The drawing under review shows one solid part. Ordinate dimensions are in mm from its lowest x, y, z. Round coordinates to 2 decimals unless told otherwise and drop trailing zeros. Order: outer loops, then holes, each group sorted by start corner. A loop starts at its lowest first (then second) coordinate and runs counter-clockwise, first axis right, second up. Notation, with made-up numbers: M 81.5,13 L 139.5,13 A14 cw 139.5,28 Z; hole C -29.5,-25 d5. An arc over 180 degrees is marked long. Answer as a JSON object with one key per item and string values. Group by question number.
1) Consider section D-D, the plane x = 7. Write out the cut boundary in (y, z) (1 decimal).
2) Consider section A-A, the plane x = 70.5. Write out the cut boundary in (y, z).
3) Insertion check: pin 1 Ø4 at (x, z) = (15.5, 69) entering from -Y; pin 2 Ø6.5 at (x, y) = (71.5, 7) entering from +Z; pin 3 Ø2 at (x, y) = (33.5, 3) entering from +Z (1 decimal); pin 4 Ø1 at (x, y) = (8.5, 5) entering from -Z. Each pin has a flat end and moves straight along its axis. Give the tip position at first contact, or say it passes through.
4) To check wall thickness, follow line 1 (Y direction, x = 1.1, z = 70.5); line 2 (Y direction, x = 70.5, z = 1.9); line 3 (Z direction, x = 73.5, y = 8). State the ranges of each line that lie inside material, in increasing order.
5) Consider section C-C, the plane y = 10.25. Write out the cut boundary in (x, z).
6) Consider section B-B, the plane z = 70.5. Write out the cut boundary in (x, y), then the cut area to 3 significant figures.
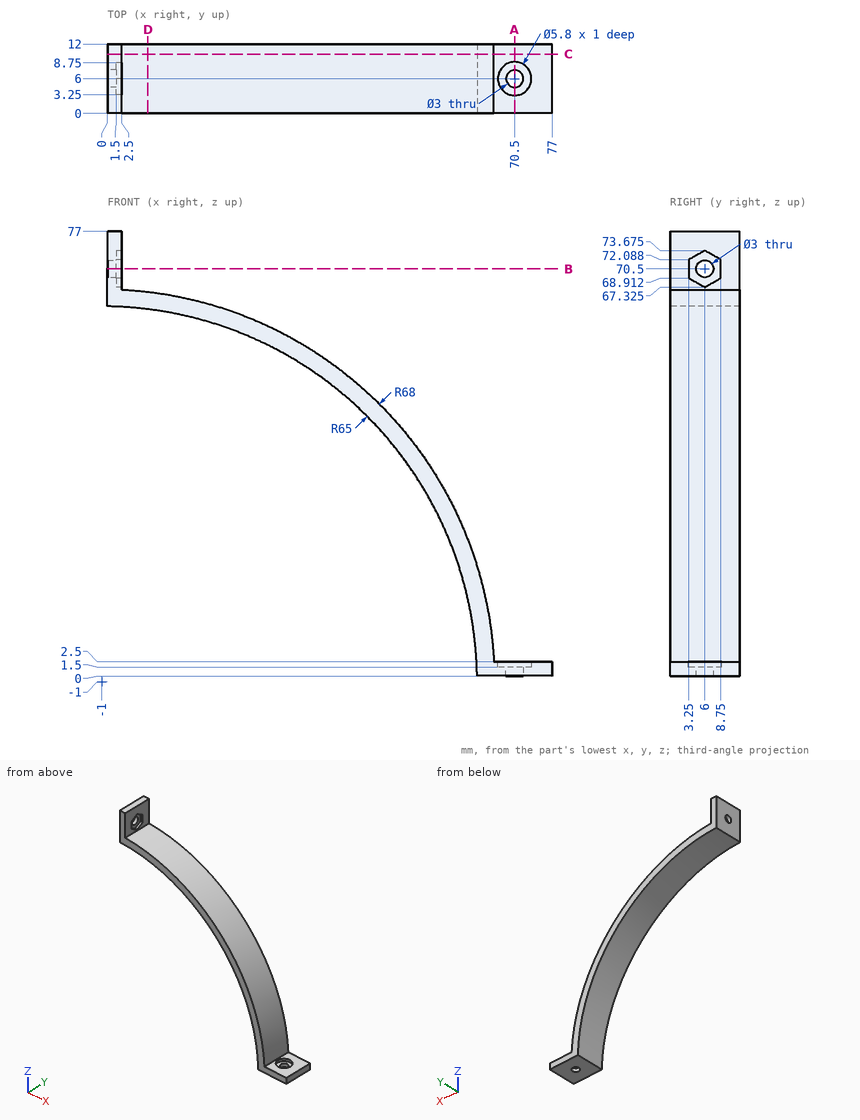
Results list:
{
 "1": {"outline": "M 0,63.5 L 12,63.5 L 12,66.5 L 0,66.5 Z"},
 "2": {"outline": "M 0,0 L 4.5,0 L 4.5,1.5 L 3.1,1.5 L 3.1,2.5 L 0,2.5 Z; M 7.5,0 L 12,0 L 12,2.5 L 8.9,2.5 L 8.9,1.5 L 7.5,1.5 Z"},
 "3": {"pin 1": "through", "pin 2": "z = 2.5", "pin 3": "z = 58.2", "pin 4": "z = 63.23"},
 "4": {"line 1": "0 to 4.5, 7.5 to 12", "line 2": "0 to 3.1, 8.9 to 12", "line 3": "0 to 2.5"},
 "5": {"outline": "M 0,63.99 A65 cw 63.99,0 L 77,0 L 77,2.5 L 66.91,2.5 A68 ccw 2.5,66.91 L 2.5,77 L 0,77 Z"},
 "6": {"outline": "M 0,0 L 2.5,0 L 2.5,3.25 L 1.5,3.25 L 1.5,4.5 L 0,4.5 Z; M 0,7.5 L 1.5,7.5 L 1.5,8.75 L 2.5,8.75 L 2.5,12 L 0,12 Z", "area": "20.0 mm^2"}
}
